Could you check a few things on this drawing? It's one solid part, dimensions in mm from its lowest x, y, z. A direction names the side the tool comes from. Round coordinates to 2 decimals unless told otherwise and drop trailing zeros. Write each loop counter-clockwise with the first axis right and the second up, starting at its lowest first coordinate (ties: lowest second). Pieces come first, ordered by that corner, then holes. Notation, with made-up numbers: M 56,51.5 L 114,51.5 A27 cw 114,69.5 Z; hole C 83,30 d8. An arc over 180 degrees is marked long. One line per item, written item: value. Start each with the question number.
(1) I want a section at C-C on y = 7.5. Please give me the cut outline in (x, z), and give its area (3 significant figures).
(2) Which directions (+Z, -Z, +X, -X, +Y, -Y) give clear straight access to the entire face, cutting with the end or side of a thin tool? Please do the marked faces 1, 2 and 3.
(3) I want a section at B-B on x = 15. Please give me the cut outline in (y, z) (1 decimal), and give its area (3 significant figures).
(4) If I drill on L1, parallel to Z at x = 8, y = 2; L2, parallel to X at y = 8.5, z = 2.5 (1 decimal); L3, parallel to X at y = 1.25, z = 3.25 (1 decimal), over which ranges is the centre line in solid material (lowest first)?
(5) Thinking about a two-plate mould opening in Z: for the marked faces 4, 5, 6 and 7, which applies, released by +Z, released by -Z, zero draft, split by the parting line, or undercut?
(6) I'm going to push flat-ended pins straight in: pin 1 Ø9 at (x, z) = (8, 7.5) entering from -Y; pin 2 Ø2 at (x, z) = (8, 8) entering from +Y; pin 3 Ø4 at (x, z) = (23.5, 12.5) entering from +Y. Where does each tip first touch, or does it pass through?
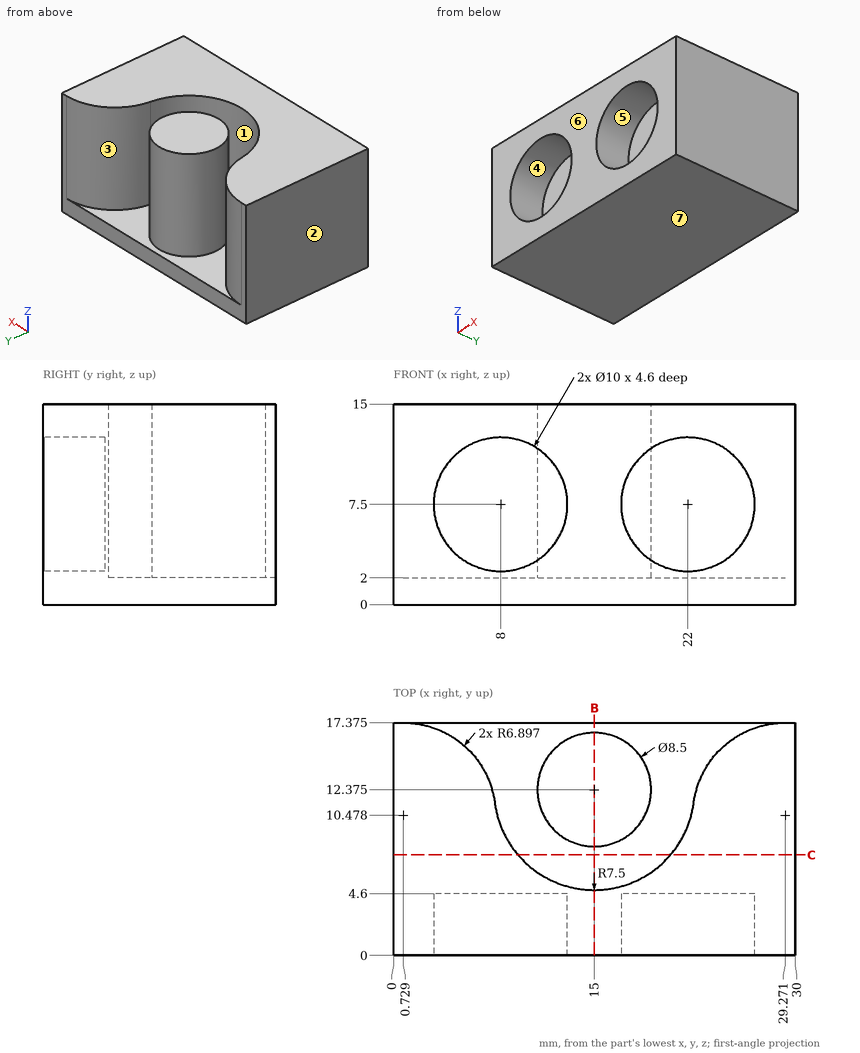
Found:
1. outline: M 0,0 L 30,0 L 30,15 L 20.7,15 L 20.7,2 L 9.3,2 L 9.3,15 L 0,15 Z
1. area: 302 mm²
2. face 1: +Z
2. face 2: +Z, -Z, -X, +Y, -Y
2. face 3: +Z, +Y
3. outline: M 0,0 L 17.4,0 L 17.4,2 L 16.6,2 L 16.6,15 L 8.1,15 L 8.1,2 L 4.9,2 L 4.9,15 L 0,15 Z
3. area: 209 mm²
4. L1: z = 0 to 2.5, 12.5 to 15
4. L2: x = 0 to 8.6, 13.3 to 16.7, 21.4 to 30
4. L3: x = 0 to 5.4, 10.6 to 19.4, 24.6 to 30
5. face 4: undercut
5. face 5: undercut
5. face 6: zero draft
5. face 7: released by -Z
6. pin 1: stops at y = 4.6
6. pin 2: stops at y = 13.35
6. pin 3: stops at y = 16.25
